Read the model definition and answer for the solid it produces. Units are mm, in the model's axes. Face numbers are marked on the shaded views. A direction names the side the tool comes from. Give positions to 0.01 mm unless a question says otherwise; leave off trailing zeros. Loops run counter-clockwise (first coordinate to the right, second up) from the corner with the lowest first, then second, coordinate; pieces in that order, holes last. Notation, with made-up numbers: (14.5, -35.75) - (22.5, -35.75) arc R36 ccw to (22.5, 0.25) - close; hole circle Ø10 at (60, 19.25). An arc over 180 degrees is marked (long way). Use a Markdown table: item, result. Add a question column.
Item 1: Which of the six approach directions +Z, -Z, +X, -X, +Y, -Y give full straight-line access (tool end or side, diameter ignored) to the marked faces 1, 2 and 3?
Item 2: This flat-tipped pin is pushed along its axis until it touches: P1, Ø1.4, axis at x = 10.5, y = 4, coming from the +Z side. Where does it stop, or does it pass through?
Item 3: A cutting plane is placed at A-A (x = 0). Determine the outline of the cut face in (y, z), plus the area to 3 significant figures.
Item 4: For a pull along Z with two mould halves and no side action, classify the marked faces 4, 5 and 6 as +Z half, -Z half, draft (parallel to the pull), parting line (faces both ways), or undercut.
Item 5: Consider probe 1 along X at (y, z) = (0, 3.25); probe 2 along Y at (x, z) = (0, 4.25); probe 3 along X at (y, z) = (-2.75, 10.25). Determine where each line is inside the solid, lowest interval first. Write a range as [from, to].
Item 6: A cutting plane is placed at D-D (z = 5). Determine the outline of the cut face in (x, y), plus the area to 3 significant figures.
Item 7: A cutting plane is placed at B-B (y = 0). Determine the outline of the cut face in (x, z), plus the area to 3 significant figures.
Item 8: A cutting plane is placed at C-C (z = 9.25). Determine the outline of the cut face in (x, y).
from build123d import *

# Parameters (mm, degrees)
PAD002_DEPTH        = 27.5
SKETCH005_W         = 1.1
SKETCH005_H         = 25
POCKET001_DEPTH     = 15.001
HOLE001_D           = 6
HOLE001_DEPTH       = 25
HOLE001_CSINK_D     = 11.2
HOLE001_CSINK_ANGLE = 90
CHAMFER_SIZE        = 0.5


with BuildPart() as part:
    # Sketch004 → Pad002 (new body, symmetric)
    with BuildSketch(Plane.YZ):
        Polygon((-7.5, 0), (7.5, 0), (7.5, 8.5), (2.806069, 8.5), (4.30718, 11.1), (-4.30718, 11.1), (-2.806069, 8.5), (-7.5, 8.5), align=None)
    extrude(amount=PAD002_DEPTH, both=True)

    # Sketch005 (on Face8 of Pad002) → Pocket001 (cut, through all)
    with BuildSketch(Plane(origin=(0, -7.5, 0), x_dir=(0, 0, -1), z_dir=(0, -1, 0))):
        with Locations((-10.55, 0)):
            Rectangle(SKETCH005_W, SKETCH005_H)
    extrude(amount=-POCKET001_DEPTH, mode=Mode.SUBTRACT)

    # Hole001
    with Locations(Plane(origin=(0, 0, 10), x_dir=(0, -1, 0), z_dir=(0, 0, 1))):
        with Locations((0, 0)):
            CounterSinkHole(HOLE001_D / 2, HOLE001_CSINK_D / 2, depth=HOLE001_DEPTH, counter_sink_angle=HOLE001_CSINK_ANGLE)

    # Chamfer
    chamfer_edges = [part.edges().sort_by_distance(p)[0] for p in [
        (27.5, 0, 0),
        (27.5, 7.5, 4.25),
        (27.5, 5.153034, 8.5),
        (27.5, 3.556624, 9.8),
        (27.5, 0, 11.1),
        (27.5, -3.556624, 9.8),
        (27.5, -5.153034, 8.5),
        (27.5, -7.5, 4.25),
        (0, -7.5, 0),
        (-27.5, 0, 0),
        (0, 7.5, 0),
        (0, -3, 0),
        (-27.5, 7.5, 4.25),
        (-27.5, 5.153034, 8.5),
        (-27.5, 3.556624, 9.8),
        (-27.5, 0, 11.1),
        (-27.5, -3.556624, 9.8),
        (-27.5, -5.153034, 8.5),
        (-27.5, -7.5, 4.25),
    ]]
    chamfer(chamfer_edges, length=CHAMFER_SIZE)


solid = part.part
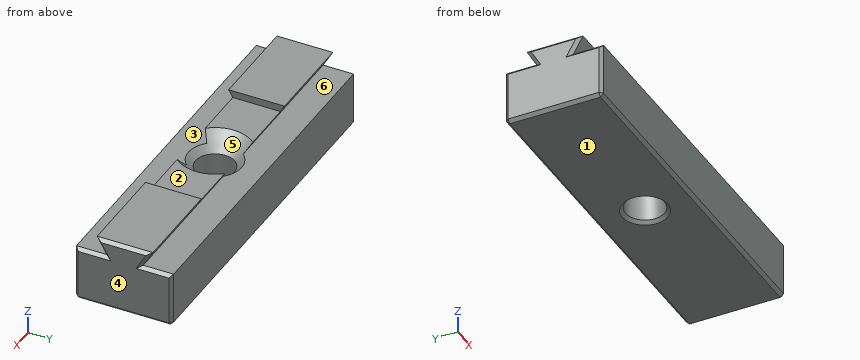
Geometry says:
| question | item | result |
|---|---|---|
| 1 | face 1 | -Z, +X, -X, +Y, -Y |
| 1 | face 2 | +Z, +Y, -Y |
| 1 | face 3 | +X, -X, -Y |
| 2 | P1 | z = 10 |
| 3 | outline | (-7.5, 0.5) - (-7, 0) - (-3.5, 0) - (-3, 0.5) - (-3, 7.4) - (-4.1, 8.5) - (-7.5, 8.5) - close; (3, 0.5) - (3.5, 0) - (7, 0) - (7.5, 0.5) - (7.5, 8.5) - (4.1, 8.5) - (3, 7.4) - close |
| 3 | area | 74.8 mm² |
| 4 | face 4 | draft |
| 4 | face 5 | +Z half |
| 4 | face 6 | undercut |
| 5 | probe 1 | [-27.5, -3], [3, 27.5] |
| 5 | probe 2 | [-7.5, -3], [3, 7.5] |
| 5 | probe 3 | [-27.5, -12.5], [12.5, 27.5] |
| 6 | outline | (-27.5, -7) - (-27, -7.5) - (27, -7.5) - (27.5, -7) - (27.5, 7) - (27, 7.5) - (-27, 7.5) - (-27.5, 7) - close; hole circle Ø6 at (0, 0) |
| 6 | area | 796 mm² |
| 7 | outline | (-27.5, 0.5) - (-27, 0) - (-3.5, 0) - (-3, 0.5) - (-3, 7.4) - (-5.6, 10) - (-12.5, 10) - (-12.5, 11.1) - (-27, 11.1) - (-27.5, 10.6) - close; (3, 0.5) - (3.5, 0) - (27, 0) - (27.5, 0.5) - (27.5, 10.6) - (27, 11.1) - (12.5, 11.1) - (12.5, 10) - (5.6, 10) - (3, 7.4) - close |
| 7 | area | 515 mm² |
| 8 | outline | (-27.5, -2.66) - (-27, -3.24) - (-3.61, -3.24) arc R4.85 cw to (-3.61, 3.24) - (-27, 3.24) - (-27.5, 2.66) - close; (3.61, -3.24) - (27, -3.24) - (27.5, -2.66) - (27.5, 2.66) - (27, 3.24) - (3.61, 3.24) arc R4.85 cw to start |
